Geometry check sheet. Reference: the model listing, model coordinates, mm. Face numbers are marked on the shaded views. A direction names the side the tool comes from. Round coordinates to 2 decimals unless told otherwise and drop trailing zeros. Order: outer loops, then holes, each group sorted by start corner. A loop starts at its lowest first (then second) coordinate and runs counter-clockwise, first axis right, second up. Notation, with made-up numbers: (45.5, -10.75) - (51.5, -10.75) arc R33 ccw to (51.5, 25.25) - close; hole circle Ø8 at (-26.75, 87.25). An arc over 180 degrees is marked (long way). One line per question, with ' | ' between items. Start each with the question number.
Q1. Sectioned sample at B-B, the plane z = -30. Enter the section's corners in (x, y).
Q2. Gauge pin test, flat ends, axial feed: P1, Ø6, axis at y = 24, z = -33.5, coming from the -X side; P2, Ø6, axis at y = 23.5, z = -9.5, coming from the +X side; P3, Ø5, axis at x = -13, z = -50, coming from the -Y side. Record the tip position at first contact, or that the pin passes through.
Q3. Tool access check on the marked faces 1, 2 and 3. Record the directions out of +Z, -Z, +X, -X, +Y, -Y that give a thin tool (end or side, any length) a straight path to the whole face; none if there is none.
Q4. Mould release check, pull along X, two halves, no side actions. Record for the marked faces 4, 5, 6 and 7: +X half, -X half, draft (parallel to the pull), parting line (faces both ways), or undercut.
Q5. Sectioned sample at C-C, the plane y = 59. Enter the section's corners in (x, z).
Q6. Sectioned sample at A-A, the plane x = 0. Enter the section's corners in (y, z), then the cut area to 3 significant figures.
Q7. Sectioned sample at D-D, the plane z = -8. Enter the section's corners in (x, y), then the cut area to 3 significant figures.
Q8. Material ranges on line 1 along Z through (x, y) = (0, 41); line 2 along X through (y, z) = (47.5, -7); line 3 along X through (y, z) = (26, -22.5), recorded low to high.
Autodesk Inventor part; units mm, degrees
ref_plane "YZ Plane" through (0, 0, 0) normal (1, 0, 0) x (0, 1, 0)
ref_plane "XZ Plane" through (0, 0, 0) normal (0, 1, 0) x (-1, 0, 0)
sketch "Эскиз1" plane through (0, 0, 0) normal (0, 0, 1) x (1, 0, 0)
  line L0 (-60, 0) -> (-60, 20)
  line L1 (-60, 20) -> (-40, 20)
  line L2 (-40, 20) -> (-40, 80)
  line L3 (-40, 80) -> (-30, 80)
  line L4 (-30, 0) -> (-20, 30)
  line L5 (-20, 30) -> (20, 30)
  line L6 (30, 0) -> (20, 30)
  line L7 (-60, 0) -> (-30, 0)
  line L8 (60, 0) -> (60, 20)
  line L9 (60, 20) -> (40, 20)
  line L10 (40, 20) -> (40, 80)
  line L11 (40, 80) -> (30, 80)
  line L12 (30, 0) -> (20, 30)
  line L13 (20, 30) -> (-20, 30)
  line L14 (60, 0) -> (30, 0)
  arc A0 (-30, 80) -> (30, 80) centre (0, 80) ccw
  point P0 (0, 0)
extrude "Выдавливание1" add sketch "Эскиз1" against normal blind 60
sketch "Эскиз3" plane through (0, 0, 0) normal (0, 1, 0) x (-1, 0, 0)
  line L0 (-20, -60) -> (20, -60)
  circle A0 centre (0, -30) radius 15
  point P0 (0, 0)
  dimension "d16" = 30
extrude "Выдавливание2" cut sketch "Эскиз3" along normal mid plane 1000
ref_plane "РабПлоскость1" through (0, 0, -30) normal (0, 0, 1) x (1, 0, 0)
sketch "Эскиз4" plane through (0, 0, -30) normal (0, 0, 1) x (1, 0, 0)
  line L0 (60, 0) -> (60, 20)
  line L1 (40, 80) -> (30, 80)
  line L2 (0, 0) -> (0, 80)
  line L3 (-60, 20) -> (-40, 80)
  line L4 (-60, 0) -> (-60, 20)
  line L5 (-60, 20) -> (-40, 20)
  line L6 (-40, 20) -> (-40, 80)
  line L7 (-40, 20) -> (-40, 80)
  line L8 (60, 20) -> (40, 80)
  line L9 (60, 20) -> (40, 20)
  line L10 (40, 20) -> (40, 80)
extrude "Выдавливание3" add sketch "Эскиз4" along normal mid plane 10
properties part number "ПЧ2021"
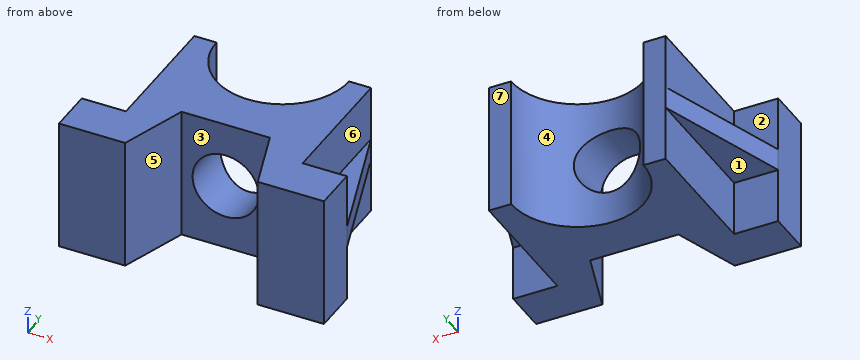
Determined:
1) outline: (-60, 0) - (-30, 0) - (-20, 30) - (-15, 30) - (-15, 54.02) arc R30 cw to (-30, 80) - (-40, 80) - (-60, 20) - close; (15, 30) - (20, 30) - (30, 0) - (60, 0) - (60, 20) - (40, 80) - (30, 80) arc R30 cw to (15, 54.02) - close
2) P1: stops at x = -59.67 | P2: stops at x = 40 | P3: stops at y = 30
3) face 1: -Z, -X, +Y | face 2: +Z, -X, +Y | face 3: +Z, -Z, -Y
4) face 4: undercut | face 5: undercut | face 6: +X half | face 7: draft
5) outline: (-47, -35) - (-40, -35) - (-40, -60) - (-21.42, -60) - (-21.42, 0) - (-40, 0) - (-40, -25) - (-47, -25) - close; (21.42, -60) - (40, -60) - (40, -35) - (47, -35) - (47, -25) - (40, -25) - (40, 0) - (21.42, 0) - close
6) outline: (30, -60) - (50, -60) - (50, -45) - (30, -45) - close; (30, -15) - (50, -15) - (50, 0) - (30, 0) - close | area: 600 mm2
7) outline: (-60, 0) - (-30, 0) - (-20, 30) - (20, 30) - (30, 0) - (60, 0) - (60, 20) - (40, 20) - (40, 80) - (30, 80) arc R30 cw to (-30, 80) - (-40, 80) - (-40, 20) - (-60, 20) - close | area: 4,290 mm2
8) line 1: z = -60 to -45, -15 to 0 | line 2: x = -40 to 40 | line 3: x = -40 to -21.33, 21.33 to 40
